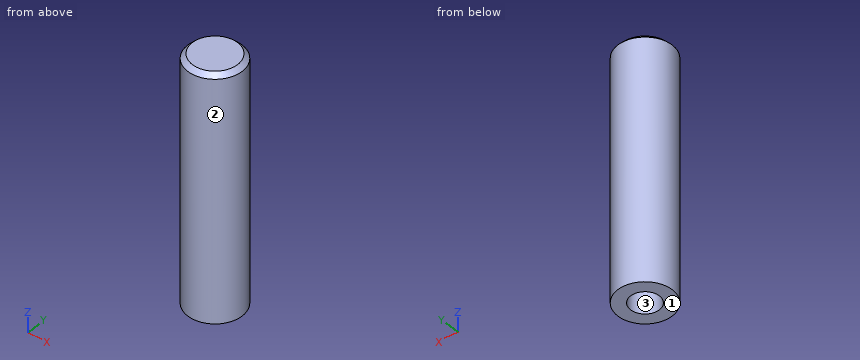
```python
from build123d import *

# Parameters (mm, degrees)
F_3_1_3_175_DURCHMESSER_BOHRUNG1_D     = 3.175
F_3_1_3_175_DURCHMESSER_BOHRUNG1_DEPTH = 10
F_3_1_3_175_DURCHMESSER_BOHRUNG1_TIP   = 0.953866233
FASE1_SIZE                             = 0.5


with BuildPart() as part:
    # Skizze1 → Rotation1 (revolve)
    with BuildSketch(Plane(origin=(78.75, 0, 0), x_dir=(0, 0, -1), z_dir=(1, 0, 0)), mode=Mode.PRIVATE) as rotation1_sk:
        Polygon((-2, 3), (-2, 0), (-22, 0), (-29, 0), (-29, 3), (-22, 3), align=None)
    revolve(rotation1_sk.sketch.rotate(Axis((78.75, 0, 22), (0, 0, -1)), 180), axis=Axis((78.75, 0, 22), (0, 0, -1)))

    # Ø3.1 (3.175) Durchmesser Bohrung1
    with Locations(Plane(origin=(0, 0, 2), x_dir=(-1, 0, 0), z_dir=(0, 0, -1))):
        with Locations((-78.75, 0)):
            Hole(F_3_1_3_175_DURCHMESSER_BOHRUNG1_D / 2, depth=F_3_1_3_175_DURCHMESSER_BOHRUNG1_DEPTH)
            with Locations((0, 0, -(F_3_1_3_175_DURCHMESSER_BOHRUNG1_DEPTH + F_3_1_3_175_DURCHMESSER_BOHRUNG1_TIP / 2))):  # 118° drill point
                Cone(0, F_3_1_3_175_DURCHMESSER_BOHRUNG1_D / 2, F_3_1_3_175_DURCHMESSER_BOHRUNG1_TIP, mode=Mode.SUBTRACT)

    # Fase1
    fase1_edges = [part.edges().sort_by_distance(p)[0] for p in [
        (78.75, 3, 29),
    ]]
    chamfer(fase1_edges, length=FASE1_SIZE)


solid = part.part
```
Geometry: final body of the model. Coordinates: model frame, mm. Face numbers are marked on the shaded views. Round coordinates to 2 decimals unless told otherwise and drop trailing zeros. Order: outer loops, then holes, each group sorted by start corner. A loop starts at its lowest first (then second) coordinate and runs counter-clockwise, first axis right, second up. Notation, with made-up numbers: M 46.5,81.5 L 102.5,81.5 A30 cw 102.5,110.5 Z; hole C -3,58.5 d3. An arc over 180 degrees is marked long. Use one line per item in the form item = value. Start each with the question number.
Q1. Cut plane B-B (z = 16). Return loops of the section in (x, y), and give its area (3 significant figures).
Q2. Mould query, pull axis Y, two halves, no side actions, for the marked faces 1, 2 and 3. Classes: +Y half, -Y half, draft (parallel to the pull), parting line (faces both ways), or undercut.
Q3. Material intervals for line 1 (Y direction, x = 78.75, z = 6.25); line 2 (X direction, y = 0, z = 9); line 3 (Y direction, x = 79.15, z = 11.25), sorted ascending. Write a range as [from, to].
Geometry results:
q1.outline = C 78.75,0 d6
q1.area = 28.3 mm^2
q2.face_1 = draft
q2.face_2 = parting line
q2.face_3 = undercut
q3.line_1 = [-3, -1.59], [1.59, 3]
q3.line_2 = [75.75, 77.16], [80.34, 81.75]
q3.line_3 = [-2.97, -1.54], [1.54, 2.97]
